Work out the finished part from the listing and answer in its coordinate system (mm). A direction names the side the tool comes from. Give positions to 0.01 mm unless a question says otherwise; leave off trailing zeros. Loops run counter-clockwise (first coordinate to the right, second up) from the corner with the lowest first, then second, coordinate; pieces in that order, holes last. Notation, with made-up numbers: (-18.75, -33) -> (15.25, -33) arc R33 ccw to (15.25, -1) -> close; hole circle Ø4 at (37, -39.5). An arc over 180 degrees is marked (long way). Answer as CSV lines item,"result". Start each with the question number.
1. Find section B-B, the plane x = -4. Give the vertices of the cut face in (y, z).
2. Determine the mould class of faces 3 (the face through (0, 6, 2)), 4 (the face through (1.4, 2.4, 2.3)), 5 (the face through (6, 0, 2)) for opening direction X: +X half, -X half, draft (parallel to the pull), parting line (faces both ways), or undercut.
3. Find the intervals of material crossed by line 1 along Y through (x, z) = (-1, 3.85); line 2 along X through (y, z) = (-1.25, 0.7); line 3 along X through (y, z) = (4.25, 4.35), in increasing order.
4. Find section D-D, the plane y = 4.75. Give the vertices of the cut face in (x, z).
5. Find section C-C, the plane z = 2. Count the separate pieces of the cut face and the enclosed holes in it, and give its area (3 significant figures).
6. Find section A-A, the plane y = -1. Give the vertices of the cut face in (x, z).
7. Flat-ended cylindrical pins translate along their axes: pin 1 Ø3.5 at (x, y) = (-3, -2.5) entering from -Z; pin 2 Ø1.9 at (x, y) = (-0.5, 0.5) entering from -Z. Find the tip coordinate at first contact, or state that the pin passes through.
8. A tool of negligible diameter and unlimited length cuts with its end or side. For faces 1 (the face through (-3, 5, 2)), 2 (the face through (-2.4, -0.2, 0)), from which of +Z, -Z, +X, -X, +Y, -Y can it reach the whole face along a straight path? Write none if from no direction.
from build123d import *

# Parameters (mm, degrees)
F0_W     = 12
F0_H     = 12
F1_DEPTH = 5.5
F2_T     = -1
F3_W     = 1
F3_H     = 3
F4_DEPTH = 4.5
F6_W     = 1.3
F6_H     = 1.2
F6_W_2   = 1.2
F6_H_2   = 1.3
F7_DEPTH = 1.4
F8_R     = 0.5


with BuildPart() as f1:
    # F0 (on Top) → F1 (new body)
    with BuildSketch(Plane.XY):
        Rectangle(F0_W, F0_H)
    extrude(amount=F1_DEPTH)

    # F2
    f2_openings = [f1.faces().sort_by_distance(p)[0] for p in [
        (0, 0, 0),
    ]]
    offset(amount=F2_T, openings=f2_openings)

    # F3 (on face) → F4 (join, through all)
    with BuildSketch(Plane(origin=(0, 0, 4.5), x_dir=(1, 0, 0), z_dir=(0, 0, -1))):
        with Locations((2.4, 0.1532564508)):
            Rectangle(F3_W, F3_H)
        Polygon((0.6, 2.9), (0.6, 5), (0, 5), (-0.6, 5), (-0.6, 2.9), (-1.4, 2.9), (-1.4, 1.9), (0, 1.9), (1.4, 1.9), (1.4, 2.9), align=None)
        with Locations((-2.4, 0.1532564508)):
            Rectangle(F3_W, F3_H)
        Polygon((0, -1.9), (-1.4, -1.9), (-1.4, -2.9), (-0.6, -2.9), (-0.6, -5), (0, -5), (0.6, -5), (0.6, -2.9), (1.4, -2.9), (1.4, -1.9), align=None)
    extrude(amount=F4_DEPTH)

    # F6 (on face) → F7 (join, through all)
    with BuildSketch(Plane(origin=(0, 0, 4.5), x_dir=(1, 0, 0), z_dir=(0, 0, -1))):
        with Locations((1.25, 0)):
            Rectangle(F6_W, F6_H)
        Rectangle(F6_W_2, F6_H)
        with Locations((0, 1.25)):
            Rectangle(F6_W_2, F6_H_2)
        with Locations((-1.25, 0)):
            Rectangle(F6_W, F6_H)
        with Locations((0, -1.25)):
            Rectangle(F6_W_2, F6_H_2)
    extrude(amount=F7_DEPTH)

    # F8
    f8_edges = [f1.edges().sort_by_distance(p)[0] for p in [
        (6, 0, 5.5),
        (0, 6, 5.5),
        (-6, 0, 5.5),
        (0, -6, 5.5),
        (-6, 6, 2.75),
        (-6, -6, 2.75),
        (6, -6, 2.75),
        (6, 6, 2.75),
    ]]
    fillet(f8_edges, radius=F8_R)


solid = f1.part
Resolved:
1,outline,"(-6, 0) -> (-5, 0) -> (-5, 4.5) -> (5, 4.5) -> (5, 0) -> (6, 0) -> (6, 5) arc R0.5 ccw to (5.5, 5.5) -> (-5.5, 5.5) arc R0.5 ccw to (-6, 5) -> close"
2,face 3,"draft"
2,face 4,"undercut"
2,face 5,"+X half"
3,line 1,"y = -6 to -5, -2.9 to -1.9, -0.6 to 0.6, 1.9 to 2.9, 5 to 6"
3,line 2,"x = -6 to -5, -2.9 to -1.9, 1.9 to 2.9, 5 to 6"
3,line 3,"x = -6 to -5, -0.6 to 0.6, 5 to 6"
4,outline,"(-6, 0) -> (-5, 0) -> (-5, 4.5) -> (-0.6, 4.5) -> (-0.6, 0) -> (0.6, 0) -> (0.6, 4.5) -> (5, 4.5) -> (5, 0) -> (6, 0) -> (6, 5) arc R0.5 ccw to (5.5, 5.5) -> (-5.5, 5.5) arc R0.5 ccw to (-6, 5) -> close"
5,separate pieces,"3"
5,enclosed holes,"1"
5,area,"60.4 mm^2"
6,outline,"(-6, 0) -> (-5, 0) -> (-5, 4.5) -> (-2.9, 4.5) -> (-2.9, 0) -> (-1.9, 0) -> (-1.9, 4.5) -> (-0.6, 4.5) -> (-0.6, 3.1) -> (0.6, 3.1) -> (0.6, 4.5) -> (1.9, 4.5) -> (1.9, 0) -> (2.9, 0) -> (2.9, 4.5) -> (5, 4.5) -> (5, 0) -> (6, 0) -> (6, 5) arc R0.5 ccw to (5.5, 5.5) -> (-5.5, 5.5) arc R0.5 ccw to (-6, 5) -> close"
7,pin 1,"stops at z = 0"
7,pin 2,"stops at z = 3.1"
8,face 1,"-Z"
8,face 2,"-Z, +X, -X, +Y, -Y"
